Job drawing, mm, ordinate dimensions from the low corner. One solid piece. A direction names the side the tool comes from. Give positions to 0.01 mm unless a question says otherwise; leave off trailing zeros. Order: outer loops, then holes, each group sorted by start corner. A loop starts at its lowest first (then second) coordinate and runs counter-clockwise, first axis right, second up. Notation, with made-up numbers: M 70,-9 L 125,-9 A30 ccw 125,18 Z; hole C 57.25,26.25 d8. An arc over 180 degrees is marked long. Use CSV: the item, a comma, the result in double quotes. Start each with the question number.
Item 1: Two-plate mould, pull along X, no slides. Class the marked faces 3, 4, 5 and 6: pulls with the +X half, pulls with the -X half, needs draft (parallel to the pull), parting line crosses it, or undercut.
Item 2: Band-saw the part on B-B on z = 73. Write the cut outline in (x, y).
Item 3: Band-saw the part on A-A on y = 12.75. Write the cut outline in (x, z), plus the area to 3 significant figures.
Item 4: Band-saw the part on D-D on z = 38. Write the cut outline in (x, y), plus the area to 3 significant figures.
Item 5: Wall check: line 1 along X through (y, z) = (5, 18); line 2 along Z through (x, y) = (18.5, 8); line 3 along Y through (x, z) = (3.5, 58). Give the ranges that are in metal, low to high.
Item 6: Pin check, flat tips, straight feed: P1, Ø18, axis at x = 26.5, z = 61, coming from the -Y side; P2, Ø4, axis at y = 8.5, z = 19.5, coming from the -X side; P3, Ø1, axis at x = 28, y = 15, coming from the -Z side; P4, Ø8, axis at x = 18, z = 18, coming from the +Y side. Stop position of each tip, or through.
Item 7: Band-saw the part on C-C on x = 14. Write the cut outline in (y, z).
Item 8: Which spindle directions (+Z, -Z, +X, -X, +Y, -Y) get a long thin tool onto all of the face, cutting with end or side? Do the marked faces 1 and 2. Say none if no direction does.
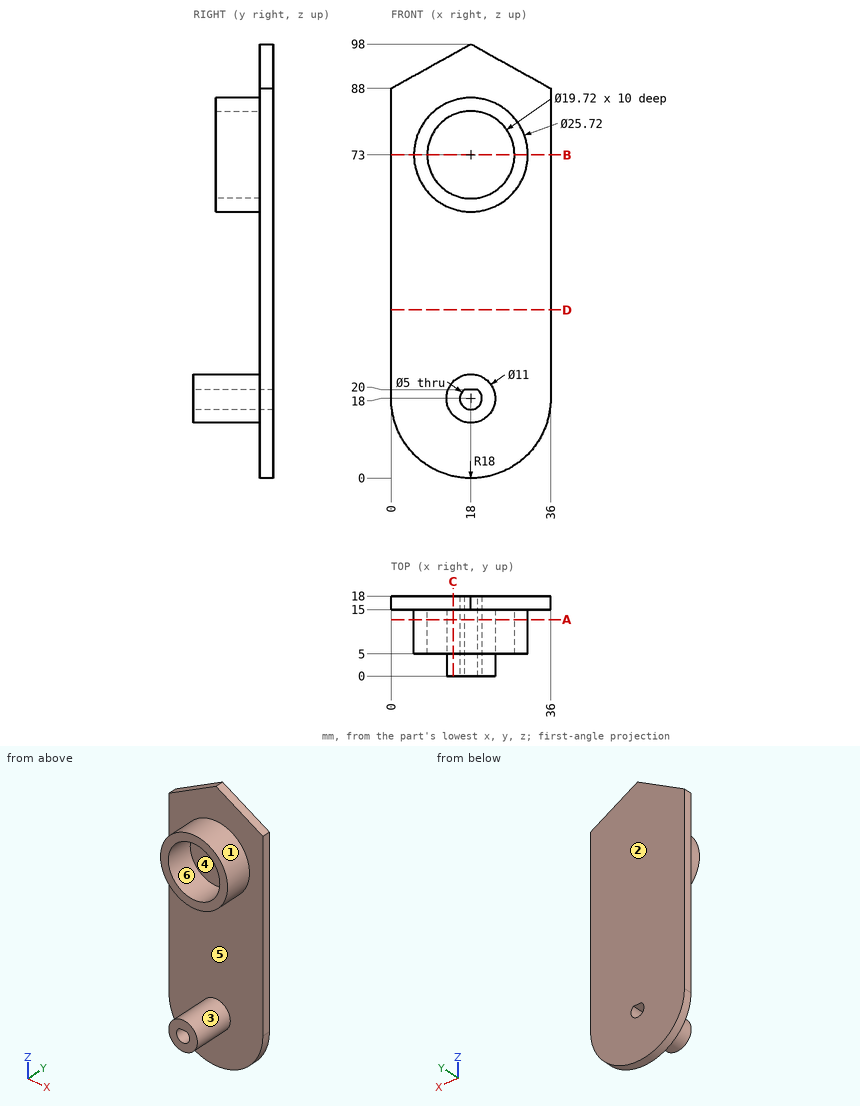
Model answer:
1,face 3,"parting line crosses it"
1,face 4,"undercut"
1,face 5,"needs draft"
1,face 6,"undercut"
2,outline,"M 0,15 L 5.14,15 L 5.14,5 L 8.14,5 L 8.14,15 L 27.86,15 L 27.86,5 L 30.86,5 L 30.86,15 L 36,15 L 36,18 L 0,18 Z"
3,outline,"C 18,73 d25.72; C 18,18 d11; hole C 18,73 d19.72; hole M 16.5,20 A2.5 ccw long 19.5,20 Z"
3,area,"291 mm^2"
4,outline,"M 0,15 L 36,15 L 36,18 L 0,18 Z"
4,area,"108 mm^2"
5,line 1,"x = 12.5 to 15.5, 20.5 to 23.5"
5,line 2,"z = 12.52 to 15.55, 20 to 23.48, 60.15 to 63.15, 82.85 to 85.85"
5,line 3,"y = 15 to 18"
6,P1,"stops at y = 5"
6,P2,"stops at x = 12.5"
6,P3,"stops at z = 2.71"
6,P4,"stops at y = 18"
7,outline,"M 0,14.23 L 15,14.23 L 15,0.45 L 18,0.45 L 18,95.78 L 15,95.78 L 15,85.22 L 5,85.22 L 5,82.01 L 15,82.01 L 15,63.99 L 5,63.99 L 5,60.78 L 15,60.78 L 15,21.77 L 0,21.77 Z"
8,face 1,"-Y"
8,face 2,"+Z, -Z, +X, -X, +Y"
